Autodesk Inventor part; units mm, degrees
ref_plane "Work Plane1" through (0, 0, 2) normal (0, 0, 1) x (1, 0, 0)
ref_plane "Work Plane2" through (0, 9.0806, 2) normal (0, 0, 1) x (1, 0, 0)
ref_plane "YZ Plane" through (0, 0, 0) normal (1, 0, 0) x (0, 1, 0)
sketch "Sketch1" plane through (0, 0, 0) normal (0, 0, 1) x (1, 0, 0)
  arc A0 (-3.9144, 3.4829) -> (-3.9144, -3.4829) centre (-6.35, 0) ccw
  arc A1 (3.9144, -3.4829) -> (3.9144, 3.4829) centre (6.35, 0) ccw
  line L0 (0, 0) -> (0, 6.6345) construction
  circle A2 centre (-6.35, 0) radius 3.6195
  line L1 (-6.35, -4.25) -> (6.35, -4.25) construction
  arc A3 (3.9144, -3.4829) -> (-3.9144, -3.4829) centre (0, -9.0806) ccw
  arc A4 (-3.9144, 3.4829) -> (3.9144, 3.4829) centre (0, 9.0806) ccw
  circle A5 centre (6.35, 0) radius 3.6195
  circle A6 centre (-6.35, 0) radius 1.75
  circle A7 centre (6.35, 0) radius 1.75
  point P0 (0, -2.25)
  point P1 (0, 2.25)
  point P2 (0, -2.25)
  dimension "d0" = 12.7
  dimension "d1" = 8.5
  dimension "d2" = 8.5
  dimension "d3" = 7.239
  dimension "d5" = 4.5
  dimension "d6" = 7.239
  dimension "d7" = 3.5
  dimension "d8" = 3.5
extrude "Extrusion1" add sketch "Sketch1" against normal blind 1 contours A4 A1 A3 A0 | A2 | A5
extrude "Extrusion2" add sketch "Sketch1" along normal blind 4 contours A2 | A5
ref_plane "Work Plane1" through (0, 0, 2) normal (0, 0, 1) x (1, 0, 0)
mirror "Mirror1" about plane through (0, 0, 2) normal (0, 0, 1) of "Extrusion1"
ref_plane "Work Plane2" through (0, 9.0806, 2) normal (0, 0, 1) x (1, 0, 0)
equation "\"d2\" = d1"
equation "\"d6\" = d3"
equation "\"d7\" = d8"
properties part number "Inner Chain"
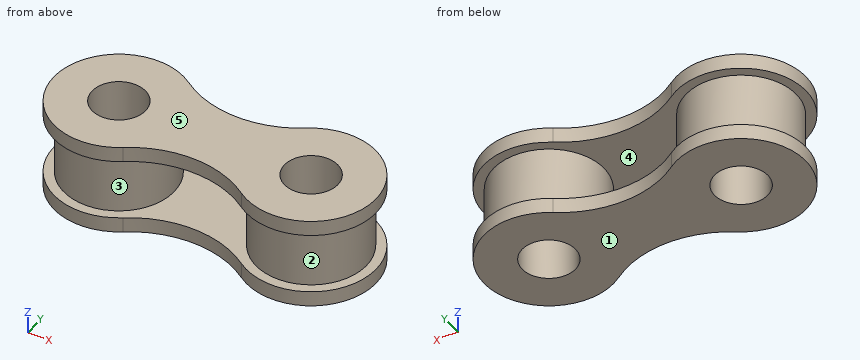
Geometry check sheet. Reference: the model listing, model coordinates, mm. Face numbers are marked on the shaded views. A direction names the side the tool comes from. Give positions to 0.01 mm unless a question says otherwise; leave off trailing zeros. Order: outer loops, then holes, each group sorted by start corner. A loop starts at its lowest first (then second) coordinate and runs counter-clockwise, first axis right, second up. Notation, with made-up numbers: (88, -4.5) - (118, -4.5) arc R22 ccw to (118, 31.5) - close; hole circle Ø7 at (84, 38). An arc over 180 degrees is marked (long way). Answer in a Markdown table with one row per item. Add a question column.
Q1. Cross-section at B-B, the plane x = -6.35. Enter the section's corners in (y, z).
Q2. Tool access check on the marked faces 4 and 5. Record the directions out of +Z, -Z, +X, -X, +Y, -Y that give a thin tool (end or side, any length) a straight path to the whole face; none if there is none.
Q3. Cross-section at D-D, the plane y = 3.25. Enter the section's corners in (x, z).
Q4. Cross-section at A-A, the plane y = 0. Enter the section's corners in (x, z).
Q5. Gauge pin test, flat ends, axial feed: pin 1 (4.5 mm diameter, centred on x = -6.35, y = 0, fed in from +Z); pin 2 (2 mm diameter, centred on x = 6.35, y = 0, fed in from +Z). Record the tip position at first contact, or that the pin passes through.
Q6. Mould release check, pull along X, two halves, no side actions. Record for the marked faces 1, 2 and 3: pulls with the +X half, pulls with the -X half, needs draft (parallel to the pull), parting line crosses it, or undercut.
Q7. Cross-section at C-C, the plane z = 0.55. Enter the section's corners in (x, y).
Q8. Material ranges on probe 1 along Y at (x, z) = (6.35, 1.95); probe 2 along X at (y, z) = (-0.75, 4.4); probe 3 along Z at (x, y) = (-9, 2.5), recorded low to high. Write a range as from..to.
Check values:
| question | item | result |
|---|---|---|
| 1 | outline | (-4.25, -1) - (-1.75, -1) - (-1.75, 5) - (-4.25, 5) - (-4.25, 4) - (-3.62, 4) - (-3.62, 0) - (-4.25, 0) - close; (1.75, -1) - (4.25, -1) - (4.25, 0) - (3.62, 0) - (3.62, 4) - (4.25, 4) - (4.25, 5) - (1.75, 5) - close |
| 2 | face 4 | none |
| 2 | face 5 | +Z, +X, -X, +Y, -Y |
| 3 | outline | (-9.09, -1) - (-3.56, -1) - (-3.56, 0) - (-4.76, 0) - (-4.76, 4) - (-3.56, 4) - (-3.56, 5) - (-9.09, 5) - (-9.09, 4) - (-7.94, 4) - (-7.94, 0) - (-9.09, 0) - close; (3.56, -1) - (9.09, -1) - (9.09, 0) - (7.94, 0) - (7.94, 4) - (9.09, 4) - (9.09, 5) - (3.56, 5) - (3.56, 4) - (4.76, 4) - (4.76, 0) - (3.56, 0) - close |
| 4 | outline | (-10.6, -1) - (-8.1, -1) - (-8.1, 5) - (-10.6, 5) - (-10.6, 4) - (-9.97, 4) - (-9.97, 0) - (-10.6, 0) - close; (-4.6, -1) - (4.6, -1) - (4.6, 5) - (-4.6, 5) - close; (8.1, -1) - (10.6, -1) - (10.6, 0) - (9.97, 0) - (9.97, 4) - (10.6, 4) - (10.6, 5) - (8.1, 5) - close; hole (-2.73, 0) - (2.73, 0) - (2.73, 4) - (-2.73, 4) - close |
| 5 | pin 1 | stops at z = 5 |
| 5 | pin 2 | passes through |
| 6 | face 1 | needs draft |
| 6 | face 2 | undercut |
| 6 | face 3 | undercut |
| 7 | outline | circle Ø7.24 at (-6.35, 0); circle Ø7.24 at (6.35, 0); hole circle Ø3.5 at (-6.35, 0); hole circle Ø3.5 at (6.35, 0) |
| 8 | probe 1 | y = -3.62..-1.75, 1.75..3.62 |
| 8 | probe 2 | x = -10.53..-7.93, -4.77..4.77, 7.93..10.53 |
| 8 | probe 3 | z = -1..0, 4..5 |
